Source: CAD feature listing. Evaluate the final solid. Frame: model axes, mm. Face numbers are marked on the shaded views. Give positions to 0.01 mm unless a question says otherwise; leave off trailing zeros. Loops run counter-clockwise (first coordinate to the right, second up) from the corner with the lowest first, then second, coordinate; pieces in that order, holes last.
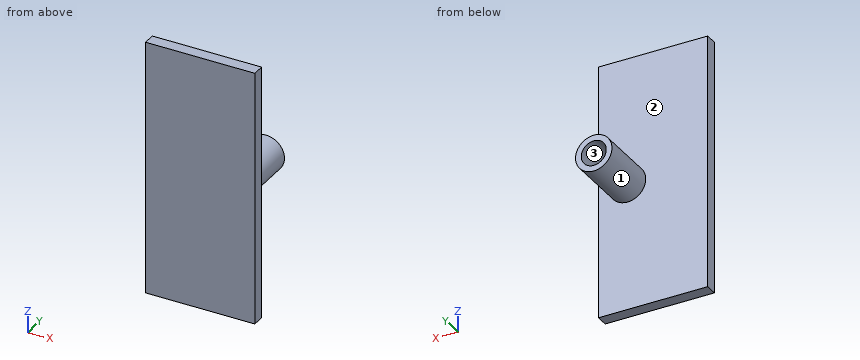
```python
from build123d import *

# Parameters (mm, degrees)
SKETCH1_W           = 45
SKETCH1_H           = 105
BOSS_EXTRUDE3_DEPTH = 5
SKETCH3_R           = 7.5
BOSS_EXTRUDE4_DEPTH = 25
SKETCH4_R           = 5.15
CUT_EXTRUDE1_DEPTH  = 20


with BuildPart() as part:
    # Sketch1 → Boss-Extrude3 (new body)
    with BuildSketch(Plane(origin=(0, 0, 0), x_dir=(1, 0, 0), z_dir=(0, 1, 0))):
        with Locations((22.5, 52.5)):
            Rectangle(SKETCH1_W, SKETCH1_H)
    extrude(amount=BOSS_EXTRUDE3_DEPTH)

    # Sketch3 → Boss-Extrude4 (add)
    with BuildSketch(Plane(origin=(0, 5, 0), x_dir=(1, 0, 0), z_dir=(0, 1, 0))):
        with Locations((33, 52.5)):
            Circle(SKETCH3_R)
    extrude(amount=BOSS_EXTRUDE4_DEPTH)

    # Sketch4 → Cut-Extrude1 (cut)
    with BuildSketch(Plane(origin=(0, 30, 0), x_dir=(1, 0, 0), z_dir=(0, 1, 0))):
        with Locations((33, 52.5)):
            Circle(SKETCH4_R)
    extrude(amount=-CUT_EXTRUDE1_DEPTH, mode=Mode.SUBTRACT)


solid = part.part
```
(1) Section C-C, the plane y = 11.75. Return the cut outline in (x, z).
A:
outline: circle Ø15 at (33, -52.5); hole circle Ø10.3 at (33, -52.5)
(2) Section D-D, the plane y = 6. Return the cut outline in (x, z), then the cut area to 3 significant figures.
A:
outline: circle Ø15 at (33, -52.5)
area: 177 mm2
(3) First-contact query: pin 1 (1.5 mm diameter, centred on x = 23.5, y = 15.5, fed in from -Z); pin 2 (8 mm diameter, centred on x = 33, z = -52.5, fed in from -Y); pin 3 (5 mm diameter, centred on x = 32.5, y = 9, fed in from -Z); pin 4 (8 mm diameter, centred on x = 39.5, y = 10.5, fed in from +Z). Flat tips, straight axial feed; report the tip coordinate or a pass-through.
A:
pin 1: passes through
pin 2: stops at y = 0
pin 3: stops at z = -60
pin 4: stops at z = -45.43
(4) Section B-B, the plane z = -52.5. Return the cut outline in (x, y), then the cut area to 3 significant figures.
A:
outline: (0, 0) - (45, 0) - (45, 5) - (40.5, 5) - (40.5, 30) - (38.15, 30) - (38.15, 10) - (27.85, 10) - (27.85, 30) - (25.5, 30) - (25.5, 5) - (0, 5) - close
area: 394 mm2
(5) Ray query, line 1 along Z through (x, y) = (33, 16.5); line 2 along X through (y, z) = (22.5, -52.5); line 3 along Y through (x, z) = (33, -64). Return the intervals inside material, ascending.
A:
line 1: z = -60 to -57.65, -47.35 to -45
line 2: x = 25.5 to 27.85, 38.15 to 40.5
line 3: y = 0 to 5
(6) Section A-A, the plane x = 33. Return the cut outline in (y, z).
A:
outline: (0, -105) - (5, -105) - (5, -60) - (30, -60) - (30, -57.65) - (10, -57.65) - (10, -47.35) - (30, -47.35) - (30, -45) - (5, -45) - (5, 0) - (0, 0) - close
(7) Mould query, pull axis X, two halves, no side actions, for the marked faces 1, 2 and 3. Classes: pulls with the +X half, pulls with the -X half, needs draft (parallel to the pull), parting line crosses it, or undercut.
A:
face 1: parting line crosses it
face 2: needs draft
face 3: undercut
